```python
from build123d import *

# Parameters (mm, degrees)
SKETCH1_W           = 46
SKETCH1_H           = 46
BOSS_EXTRUDE1_DEPTH = 5
SKETCH3_R           = 4.1
CUT_EXTRUDE2_DEPTH  = 3
SKETCH4_R           = 2.1
CUT_EXTRUDE3_DEPTH  = 6
SKETCH5_W           = 5
SKETCH5_H           = 5
BOSS_EXTRUDE2_DEPTH = 2
SKETCH6_R           = 1
CUT_EXTRUDE4_DEPTH  = 5
SKETCH7_R           = 1.6
CUT_EXTRUDE5_DEPTH  = 5


with BuildPart() as part:
    # Sketch1 → Boss-Extrude1 (new body)
    with BuildSketch(Plane(origin=(0, 0, 0), x_dir=(1, 0, 0), z_dir=(0, 1, 0))):
        Rectangle(SKETCH1_W, SKETCH1_H)
    extrude(amount=BOSS_EXTRUDE1_DEPTH)

    # Sketch3 → Cut-Extrude2 (cut)
    with BuildSketch(Plane(origin=(0, 0, 0), x_dir=(1, 0, 0), z_dir=(0, 1, 0))):
        Circle(SKETCH3_R)
    extrude(amount=CUT_EXTRUDE2_DEPTH, mode=Mode.SUBTRACT)

    # Sketch4 → Cut-Extrude3 (cut, through all)
    with BuildSketch(Plane(origin=(0, 0, 0), x_dir=(1, 0, 0), z_dir=(0, 1, 0))):
        Circle(SKETCH4_R)
    extrude(amount=CUT_EXTRUDE3_DEPTH, mode=Mode.SUBTRACT)

    # Sketch5 → Boss-Extrude2 (add)
    with BuildSketch(Plane(origin=(0, 0, 0), x_dir=(1, 0, 0), z_dir=(0, 1, 0))):
        with Locations((7.5, 0)):
            Rectangle(SKETCH5_W, SKETCH5_H)
        with Locations((-7.5, 0)):
            Rectangle(SKETCH5_W, SKETCH5_H)
    extrude(amount=-BOSS_EXTRUDE2_DEPTH)

    # Sketch6 → Cut-Extrude4 (cut)
    with BuildSketch(Plane(origin=(0, -2, 0), x_dir=(-1, 0, 0), z_dir=(0, -1, 0))):
        with Locations((7.5, 0)):
            Circle(SKETCH6_R)
        with Locations((-7.5, 0)):
            Circle(SKETCH6_R)
    extrude(amount=-CUT_EXTRUDE4_DEPTH, mode=Mode.SUBTRACT)

    # Sketch7 → Cut-Extrude5 (cut)
    with BuildSketch(Plane(origin=(0, 0, 0), x_dir=(1, 0, 0), z_dir=(0, 1, 0))):
        with Locations((-18.12, -19.125)):
            Circle(SKETCH7_R)
        with Locations((18.12, -19.125)):
            Circle(SKETCH7_R)
        with Locations((18.12, 19.125)):
            Circle(SKETCH7_R)
        with Locations((-18.12, 19.125)):
            Circle(SKETCH7_R)
    extrude(amount=CUT_EXTRUDE5_DEPTH, mode=Mode.SUBTRACT)


solid = part.part
```
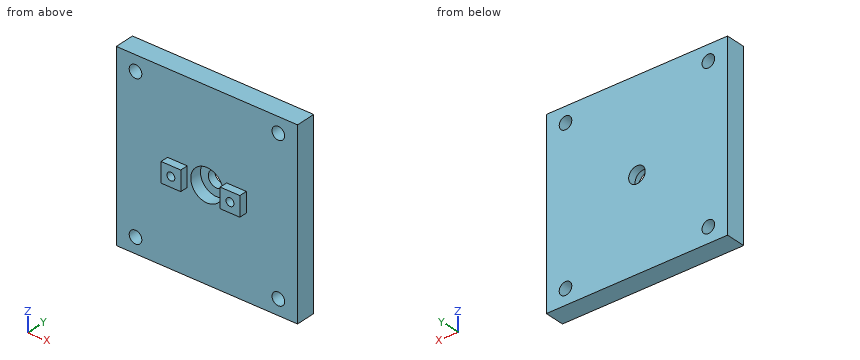
Geometry: final body of the model. Coordinates: model frame, mm. Coordinates: 2 decimals unless noted, no trailing zeros. Order: outer loops, then holes, each group sorted by start corner. A loop starts at its lowest first (then second) coordinate and runs counter-clockwise, first axis right, second up. Notation, with made-up numbers: (80, 44) - (116, 44) arc R16 cw to (116, 60) - close; hole circle Ø5 at (29, 70). An arc over 180 degrees is marked (long way). Return JSON: item names as keys, results as strings. Group by question number.
1. Cut plane B-B (z = 0). Output: boundary loops of the cut face in (x, y).
2. Pin query (flat end, axial travel): pin 1 (3.5 mm diameter, centred on x = -18.12, z = 19.125, fed in from -Y); pin 2 (1 mm diameter, centred on y = -1.5, z = -1, fed in from -X); pin 3 (0.6 mm diameter, centred on y = -1.5, z = -0.5, fed in from +X); pin 4 (2.5 mm diameter, centred on x = -18.12, z = -19.125, fed in from +Y). Return the tip coordinate at first contact, or that it passes through.
3. Material intervals for line 1 along Z through (x, y) = (18.12, 1.65) (3 decimals); line 2 along Z through (x, y) = (-7.5, 1); line 3 along X through (y, z) = (0.5, 20), sorted ascending. Write a range as [from, to].
4. Cut plane C-C (x = 0). Output: boundary loops of the cut face in (y, z).
5. Cut plane A-A (x = -18.12). Output: boundary loops of the cut face in (y, z) (3 decimals), plus the area to 3 significant figures.
6. Cut plane D-D (y = 1.5). Output: boundary loops of the cut face in (x, z) (3 decimals).
Resolved:
{
 "1": {"outline": "(-23, 0) - (-10, 0) - (-10, -2) - (-8.5, -2) - (-8.5, 3) - (-6.5, 3) - (-6.5, -2) - (-5, -2) - (-5, 0) - (-4.1, 0) - (-4.1, 3) - (-2.1, 3) - (-2.1, 5) - (-23, 5) - close; (2.1, 3) - (4.1, 3) - (4.1, 0) - (5, 0) - (5, -2) - (6.5, -2) - (6.5, 3) - (8.5, 3) - (8.5, -2) - (10, -2) - (10, 0) - (23, 0) - (23, 5) - (2.1, 5) - close"},
 "2": {"pin 1": "stops at y = 0", "pin 2": "stops at x = -10", "pin 3": "stops at x = 10", "pin 4": "passes through"},
 "3": {"line 1": "z = [-23, -20.725], [-17.525, 17.525], [20.725, 23]", "line 2": "z = [-23, -1], [1, 23]", "line 3": "x = [-23, -19.46], [-16.78, 16.78], [19.46, 23]"},
 "4": {"outline": "(0, -23) - (5, -23) - (5, -2.1) - (3, -2.1) - (3, -4.1) - (0, -4.1) - close; (0, 4.1) - (3, 4.1) - (3, 2.1) - (5, 2.1) - (5, 23) - (0, 23) - close"},
 "5": {"outline": "(0, -23) - (5, -23) - (5, -20.725) - (0, -20.725) - close; (0, -17.525) - (5, -17.525) - (5, 17.525) - (0, 17.525) - close; (0, 20.725) - (5, 20.725) - (5, 23) - (0, 23) - close", "area": "198 mm²"},
 "6": {"outline": "(-23, -23) - (23, -23) - (23, 23) - (-23, 23) - close; hole circle Ø3.2 at (-18.12, -19.125); hole circle Ø3.2 at (-18.12, 19.125); hole circle Ø2 at (-7.5, 0); hole circle Ø8.2 at (0, 0); hole circle Ø2 at (7.5, 0); hole circle Ø3.2 at (18.12, -19.125); hole circle Ø3.2 at (18.12, 19.125)"}
}
